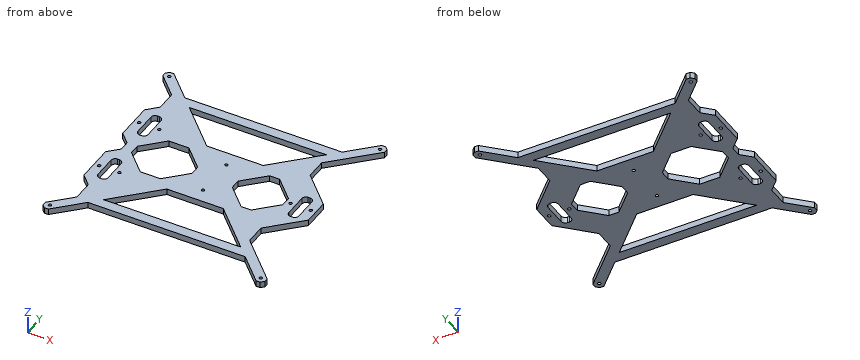
from build123d import *

# Parameters (mm, degrees)
MODEL_R                  = 1.5
RESSALTO_EXTRUS_O1_DEPTH = 6


with BuildPart() as part:
    # Model → Ressalto-extrusão1 (new body)
    with BuildSketch(Plane.XY):
        Polygon((27.223932907, 227.848775031), (25.223932907, 227.848775031), (22.223932907, 224.848775031), (22.223932907, 222.848775031), (22.223932907, 220.848775031), (42.223932907, 200.848775031), (42.223932907, 180.848775031), (32.223932907, 170.848775031), (32.223932907, 132.848775031), (42.223932907, 122.848775031), (42.223932907, 112.848775031), (32.223932907, 102.848775031), (32.223932907, 64.848775031), (42.223932907, 54.848775031), (42.223932907, 34.848775031), (22.223932907, 14.848775031), (22.223932907, 10.848775031), (25.223932907, 7.848775031), (27.223932907, 7.848775031), (29.223932907, 7.848775031), (54.223932907, 32.848775031), (210.223932907, 32.848775031), (235.223932907, 7.848775031), (237.223932907, 7.848775031), (239.223932907, 7.848775031), (242.223932907, 10.848775031), (242.223932907, 14.848775031), (222.223932907, 34.848775031), (202.223932907, 54.848775031), (202.223932907, 74.848775031), (222.223932907, 94.848775031), (232.223932907, 104.848775031), (232.223932907, 130.848775031), (222.223932907, 140.848775031), (202.223932907, 160.848775031), (202.223932907, 180.848775031), (242.223932907, 220.848775031), (242.223932907, 223.848775031), (242.223932907, 224.848775031), (239.223932907, 227.848775031), (235.223932907, 227.848775031), (212.223932907, 204.848775031), (210.223932907, 202.848775031), (54.223932907, 202.848775031), (29.223932907, 227.848775031), align=None)
        with Locations((37.223932907, 152.848775031)):
            Circle(MODEL_R, mode=Mode.SUBTRACT)
        with Locations((57.223932907, 152.848775031)):
            Circle(MODEL_R, mode=Mode.SUBTRACT)
        with Locations((37.223932907, 82.848775031)):
            Circle(MODEL_R, mode=Mode.SUBTRACT)
        with Locations((57.223932907, 82.848775031)):
            Circle(MODEL_R, mode=Mode.SUBTRACT)
        with Locations((227.223932907, 117.848775031)):
            Circle(MODEL_R, mode=Mode.SUBTRACT)
        with Locations((207.223932907, 117.848775031)):
            Circle(MODEL_R, mode=Mode.SUBTRACT)
        with Locations((27.723932907, 222.348775031)):
            Circle(MODEL_R, mode=Mode.SUBTRACT)
        with Locations((236.723932907, 13.348775031)):
            Circle(MODEL_R, mode=Mode.SUBTRACT)
        with Locations((236.723932907, 222.348775031)):
            Circle(MODEL_R, mode=Mode.SUBTRACT)
        with Locations((27.723932907, 13.348775031)):
            Circle(MODEL_R, mode=Mode.SUBTRACT)
        with Locations((132.223932907, 96.848775031)):
            Circle(MODEL_R, mode=Mode.SUBTRACT)
        with Locations((132.223932907, 137.848775031)):
            Circle(MODEL_R, mode=Mode.SUBTRACT)
        Polygon((172.223932907, 164.848775031), (170.223932907, 162.848775031), (160.223932907, 152.848775031), (104.223932907, 152.848775031), (64.223932907, 192.848775031), (200.223932907, 192.848775031), align=None, mode=Mode.SUBTRACT)
        Polygon((160.223932907, 82.848775031), (104.223932907, 82.848775031), (64.223932907, 42.848775031), (200.223932907, 42.848775031), align=None, mode=Mode.SUBTRACT)
        Polygon((52.223932907, 122.848775031), (72.223932907, 142.848775031), (92.223932907, 142.848775031), (112.223932907, 122.848775031), (112.223932907, 112.848775031), (92.223932907, 92.848775031), (72.223932907, 92.848775031), (52.223932907, 112.848775031), align=None, mode=Mode.SUBTRACT)
        Polygon((182.223932907, 142.848775031), (202.223932907, 122.848775031), (202.223932907, 112.848775031), (182.223932907, 92.848775031), (172.223932907, 92.848775031), (152.223932907, 112.848775031), (152.223932907, 122.848775031), (172.223932907, 142.848775031), align=None, mode=Mode.SUBTRACT)
        with BuildLine():
            Line((42.223932907, 71.848775031), (42.223932907, 94.848775031))
            ThreePointArc((42.223932907, 94.848775031), (43.395505782, 97.677202156), (46.223932907, 98.848775031))
            Line((46.223932907, 98.848775031), (48.223932907, 98.848775031))
            ThreePointArc((48.223932907, 98.848775031), (51.052360031, 97.677202156), (52.223932907, 94.848775031))
            Line((52.223932907, 94.848775031), (52.223932907, 71.848775031))
            ThreePointArc((52.223932907, 71.848775031), (51.052360031, 69.020347906), (48.223932907, 67.848775031))
            Line((48.223932907, 67.848775031), (46.223932907, 67.848775031))
            ThreePointArc((46.223932907, 67.848775031), (43.395505782, 69.020347906), (42.223932907, 71.848775031))
        make_face(mode=Mode.SUBTRACT)
        with BuildLine():
            Line((42.223932907, 141.855811927), (42.223932907, 164.855811927))
            ThreePointArc((42.223932907, 164.855811927), (43.395505782, 167.684239052), (46.223932907, 168.855811927))
            Line((46.223932907, 168.855811927), (48.223932907, 168.855811927))
            ThreePointArc((48.223932907, 168.855811927), (51.052360031, 167.684239052), (52.223932907, 164.855811927))
            Line((52.223932907, 164.855811927), (52.223932907, 141.855811927))
            ThreePointArc((52.223932907, 141.855811927), (51.052360031, 139.027384802), (48.223932907, 137.855811927))
            Line((48.223932907, 137.855811927), (46.223932907, 137.855811927))
            ThreePointArc((46.223932907, 137.855811927), (43.395505782, 139.027384802), (42.223932907, 141.855811927))
        make_face(mode=Mode.SUBTRACT)
        with BuildLine():
            Line((212.223932907, 105.711651424), (212.223932907, 128.711651424))
            ThreePointArc((212.223932907, 128.711651424), (213.395505782, 131.540078549), (216.223932907, 132.711651424))
            Line((216.223932907, 132.711651424), (218.223932907, 132.711651424))
            ThreePointArc((218.223932907, 132.711651424), (221.052360031, 131.540078549), (222.223932907, 128.711651424))
            Line((222.223932907, 128.711651424), (222.223932907, 105.711651424))
            ThreePointArc((222.223932907, 105.711651424), (221.052360031, 102.883224299), (218.223932907, 101.711651424))
            Line((218.223932907, 101.711651424), (216.223932907, 101.711651424))
            ThreePointArc((216.223932907, 101.711651424), (213.395505782, 102.883224299), (212.223932907, 105.711651424))
        make_face(mode=Mode.SUBTRACT)
    extrude(amount=RESSALTO_EXTRUS_O1_DEPTH)


solid = part.part
The model under review builds one solid part; all positions refer to its coordinate system, in mm. Give positions to 0.01 mm unless a question says otherwise; leave off trailing zeros. Write each loop counter-clockwise with the first axis right and the second up, starting at its lowest first coordinate (ties: lowest second). Pieces come first, ordered by that corner, then holes.
1. Wall thickness on L1, parallel to Y at x = 141.5, z = 3.8; L2, parallel to Y at x = 180, z = 4.75; L3, parallel to X at y = 139, z = 4.8: over which ranges is each line inside the solid? List them lowest first.
2. For P1, Ø1.6, axis at x = 47.5, z = 1.5, coming from the -Y side; P2, Ø2, axis at x = 217.5, z = 3, coming from the -Y side; P3, Ø1.5, axis at y = 72.5, z = 0.5, coming from the +X side; P4, Ø1.8, axis at x = 57.22, y = 152.85, coming from the +Z side, all flat-tipped, find the tip position at first contact; note any pin that passes through.
3. Add section C-C, the plane x = 164.5. Write out the cut boundary in (y, z), plus the area to 3 significant figures.
4. Add section D-D, the plane z = 0.9. Count the separate pieces of the cut face and the enclosed holes in it, plus the area to 3 significant figures.
5. Add section A-A, the plane x = 119. Write out the cut boundary in (y, z), plus the area to 3 significant figures.
6. Add section B-B, the plane y = 24.5. Write out the cut boundary in (x, z).
Worked answers:
1. L1: y = 32.85 to 42.85, 82.85 to 152.85, 192.85 to 202.85
1. L2: y = 32.85 to 42.85, 63.07 to 92.85, 142.85 to 172.62, 192.85 to 202.85
1. L3: x = 32.22 to 43.42, 51.02 to 68.38, 96.07 to 131.26, 133.19 to 168.38, 186.07 to 224.07
2. P1: stops at y = 25.32
2. P2: stops at y = 24.57
2. P3: stops at x = 202.22
2. P4: passes through
3. outline: (32.85, 0) - (42.85, 0) - (42.85, 6) - (32.85, 6) - close; (78.57, 0) - (100.57, 0) - (100.57, 6) - (78.57, 6) - close; (135.12, 0) - (157.12, 0) - (157.12, 6) - (135.12, 6) - close; (192.85, 0) - (202.85, 0) - (202.85, 6) - (192.85, 6) - close
3. area: 384 mm2
4. separate pieces: 1
4. enclosed holes: 19
4. area: 19,100 mm2
5. outline: (32.85, 0) - (42.85, 0) - (42.85, 6) - (32.85, 6) - close; (82.85, 0) - (152.85, 0) - (152.85, 6) - (82.85, 6) - close; (192.85, 0) - (202.85, 0) - (202.85, 6) - (192.85, 6) - close
5. area: 540 mm2
6. outline: (31.88, 0) - (45.88, 0) - (45.88, 6) - (31.88, 6) - close; (218.57, 0) - (232.57, 0) - (232.57, 6) - (218.57, 6) - close
